For this review, take the finished solid that the model builds, in its own axes (mm). Face numbers are marked on the shaded views. A direction names the side the tool comes from. Round coordinates to 2 decimals unless told otherwise and drop trailing zeros. Order: outer loops, then holes, each group sorted by start corner. A loop starts at its lowest first (then second) coordinate and runs counter-clockwise, first axis right, second up.
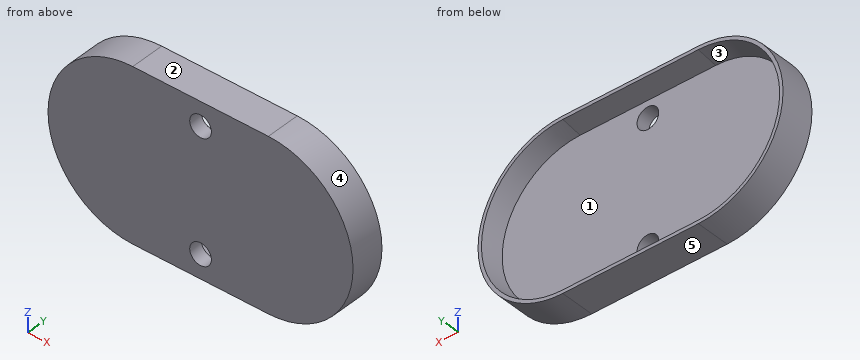
```python
from build123d import *

# Parameters (mm, degrees)
BOSS_EXTRUDE1_DEPTH = 2
BOSS_EXTRUDE2_DEPTH = 3
CHAMFER1_SIZE       = 0.5
CHAMFER1_SIZE_2     = 3
SKETCH3_R           = 1.6
CUT_EXTRUDE1_DEPTH  = 27.220221204


with BuildPart() as part:
    # Sketch1 → Boss-Extrude1 (new body)
    with BuildSketch(Plane(origin=(0, 0, 0), x_dir=(1, 0, 0), z_dir=(0, 1, 0))):
        with BuildLine():
            Line((-10, 12.5), (10, 12.5))
            ThreePointArc((10, 12.5), (22.5, 0), (10, -12.5))
            Line((10, -12.5), (-10, -12.5))
            ThreePointArc((-10, -12.5), (-22.5, 0), (-10, 12.5))
        make_face()
    extrude(amount=BOSS_EXTRUDE1_DEPTH)

    # Sketch2 → Boss-Extrude2 (add)
    with BuildSketch(Plane(origin=(0, 2, 0), x_dir=(1, 0, 0), z_dir=(0, 1, 0))):
        with BuildLine():
            Line((10, 12.5), (-10, 12.5))
            ThreePointArc((-10, 12.5), (-22.5, 0), (-10, -12.5))
            Line((-10, -12.5), (10, -12.5))
            ThreePointArc((10, -12.5), (22.5, 0), (10, 12.5))
        make_face()
        with BuildLine():
            Line((-10, -11.5), (10, -11.5))
            ThreePointArc((10, -11.5), (21.5, 0), (10, 11.5))
            Line((10, 11.5), (-10, 11.5))
            ThreePointArc((-10, 11.5), (-21.5, 0), (-10, -11.5))
        make_face(mode=Mode.SUBTRACT)
    extrude(amount=BOSS_EXTRUDE2_DEPTH)

    # Chamfer1
    # the kernel refuses this chamfer: 3, 0.5 mm, written as the material it takes off along each edge
    with BuildSketch(Plane(origin=(-10, 5, 11.5), x_dir=(0, 0.2220622368174743, 0.9750324932942593), z_dir=(1, 0, 0))) as chamfer1_piece_1_section:
        Polygon((CHAMFER1_SIZE * 0.975032493294, CHAMFER1_SIZE * 0.222062236817), (-CHAMFER1_SIZE_2 * 0.222062236817, CHAMFER1_SIZE_2 * 0.975032493294), (0, 0), align=None)
    chamfer1_piece_1 = extrude(amount=20, mode=Mode.PRIVATE)
    chamfer1_piece_1 = split(chamfer1_piece_1, bisect_by=Plane(origin=(0, 2, 11.634388756), z_dir=(0, 1, 0)), keep=Keep.TOP, mode=Mode.PRIVATE)
    add(chamfer1_piece_1, mode=Mode.SUBTRACT)
    with BuildSketch(Plane(origin=(10, 5, 0), x_dir=(0, 0, 1), z_dir=(-1, 0, 0))) as chamfer1_piece_2_section:
        Polygon((11.5 + CHAMFER1_SIZE, 0), (11.5, -CHAMFER1_SIZE_2), (11.5, 0), align=None)
    chamfer1_piece_2 = revolve(axis=Axis((10, 5, 0), (0, 1, 0)), revolution_arc=180, mode=Mode.PRIVATE)
    chamfer1_piece_2 = split(chamfer1_piece_2, bisect_by=Plane(origin=(21.727349814, 2, 0), z_dir=(0, 1, 0)), keep=Keep.TOP, mode=Mode.PRIVATE)
    add(chamfer1_piece_2, mode=Mode.SUBTRACT)
    with BuildSketch(Plane(origin=(10, 5, -11.5), x_dir=(0, 0.2220622368174743, -0.9750324932942593), z_dir=(-1, 0, 0))) as chamfer1_piece_3_section:
        Polygon((CHAMFER1_SIZE * 0.975032493294, CHAMFER1_SIZE * 0.222062236817), (-CHAMFER1_SIZE_2 * 0.222062236817, CHAMFER1_SIZE_2 * 0.975032493294), (0, 0), align=None)
    chamfer1_piece_3 = extrude(amount=20, mode=Mode.PRIVATE)
    chamfer1_piece_3 = split(chamfer1_piece_3, bisect_by=Plane(origin=(0, 2, -11.634388756), z_dir=(0, 1, 0)), keep=Keep.TOP, mode=Mode.PRIVATE)
    add(chamfer1_piece_3, mode=Mode.SUBTRACT)
    with BuildSketch(Plane(origin=(-10, 5, 0), x_dir=(0, 0, -1), z_dir=(1, 0, 0))) as chamfer1_piece_4_section:
        Polygon((11.5 + CHAMFER1_SIZE, 0), (11.5, -CHAMFER1_SIZE_2), (11.5, 0), align=None)
    chamfer1_piece_4 = revolve(axis=Axis((-10, 5, 0), (0, 1, 0)), revolution_arc=180, mode=Mode.PRIVATE)
    chamfer1_piece_4 = split(chamfer1_piece_4, bisect_by=Plane(origin=(-21.727349812, 2, 0), z_dir=(0, 1, 0)), keep=Keep.TOP, mode=Mode.PRIVATE)
    add(chamfer1_piece_4, mode=Mode.SUBTRACT)

    # Sketch3 → Cut-Extrude1 (cut, through all)
    with BuildSketch(Plane.XZ):
        with Locations(Location((0, -9, 0), (0, 0, 270))):
            Circle(SKETCH3_R)
        with Locations(Location((0, 9, 0), (0, 0, 270))):
            Circle(SKETCH3_R)
    extrude(amount=-CUT_EXTRUDE1_DEPTH, mode=Mode.SUBTRACT)


solid = part.part
```
Q1. Take a section at A-A, the plane x = 0. State the section outline as (y, z) points, plus the area to 3 significant figures.
Q2. Clearance check with flat-ended pins moving along their axes: pin 1 (10 mm diameter, centred on x = 2.5, z = -2, fed in from +Y); pin 2 (1.9 mm diameter, centred on x = 0, z = -9, fed in from +Y); pin 3 (3 mm diameter, centred on y = 4, z = 10, fed in from -X); pin 4 (1 mm diameter, centred on y = 3, z = 7, fed in from +X). State where each tip first meets the part, or that it passes through.
Q3. Tool access review of the marked faces 1 and 2: name each direction out of +Z, -Z, +X, -X, +Y, -Y from which nothing blocks a thin tool from reaching the whole face with its end or side.
Q4. Take a section at B-B, the plane y = 2.7. State the section outline as (x, z) points, plus the area to 3 significant figures.
Q5. Take a section at C-C, the plane z = 0. State the section outline as (x, y) points, plus the area to 3 significant figures.
Q6. Mouldability with a two-part tool opening along Z and no side actions: class the marked faces 3, 4 and 5 as +Z half, -Z half, draft (parallel to the pull), parting line (faces both ways), or undercut.
Q7. Wall thickness on line 1 (Y direction, x = 17.5, z = -6); line 2 (X direction, y = 1, z = 8.5); line 3 (Z direction, x = 12, y = 4.5): over which ranges is each line inside the solid? List them lowest first.
Working result:
1. outline: (0, -12.5) - (5, -12.5) - (5, -12) - (2, -11.5) - (2, -10.6) - (0, -10.6) - close; (0, -7.4) - (2, -7.4) - (2, 7.4) - (0, 7.4) - close; (0, 10.6) - (2, 10.6) - (2, 11.5) - (5, 12) - (5, 12.5) - (0, 12.5) - close
1. area: 41.7 mm2
2. pin 1: stops at y = 2
2. pin 2: passes through
2. pin 3: stops at x = -19.17
2. pin 4: stops at x = 20.68
3. face 1: +Y
3. face 2: +Z, +X, -X, +Y, -Y
4. outline: (-10, -12.5) - (10, -12.5) arc R12.5 ccw to (10, 12.5) - (-10, 12.5) arc R12.5 ccw to start; hole (-10, -11.62) - (10, -11.62) arc R11.62 ccw to (10, 11.62) - (-10, 11.62) arc R11.62 ccw to start
4. area: 102 mm2
5. outline: (-22.5, 0) - (22.5, 0) - (22.5, 5) - (22, 5) - (21.5, 2) - (-21.5, 2) - (-22, 5) - (-22.5, 5) - close
5. area: 94.5 mm2
6. face 3: undercut
6. face 4: parting line
6. face 5: -Z half
7. line 1: y = 0 to 2
7. line 2: x = -19.17 to -1.52, 1.52 to 19.17
7. line 3: z = -12.34 to -11.75, 11.75 to 12.34
